Print and shaded views of the part. All mm, measured from the part's lowest x, y and z. Give positions to 0.01 mm unless a question says otherwise; leave off trailing zeros. Write each loop counter-clockwise with the first axis right and the second up, starting at its lowest first coordinate (ties: lowest second). Pieces come first, ordered by that corner, then holes. Notation, with made-up numbers: M 51,-2 L 79,-2 A20 ccw 79,4 Z; hole C 38,18 d1. An arc over 180 degrees is marked long. One line per question, with ' | ' between items. Start each with the question number.
1. Flat gauge pins, fed straight in: pin 1 (2 mm diameter, centred on x = 26.5, y = 117.5, fed in from -Z); pin 2 (6 mm diameter, centred on y = 52, z = 161, fed in from -X); pin 3 (2 mm diameter, centred on y = 272.5, z = 48.5, fed in from -X). Where does each tip first touch, or does it go through?
2. Cut at A-A, the plane x = 10. Write the cut outline in (y, z), then the cut area to 3 significant figures.
3. Wall check: L1, parallel to X at y = 82, z = 153; L2, parallel to Y at x = 90, z = 57.5; L3, parallel to Z at x = 62.5, y = 98. Give the ranges that are in metal, low to high.
4. Pull direction X, two halves, no side cores. Call the marked faces 1, 2 and 3: released by +X, released by -X, zero draft, split by the parting line, or undercut.
5. Cut at D-D, the plane x = 48.5. Write the cut outline in (y, z), then the cut area to 3 significant figures.
6. Cut at B-B, the plane y = 252. Write the cut outline in (x, z).
7. Cut at C-C, the plane y = 144.5. Write the cut outline in (x, z) (1 decimal).
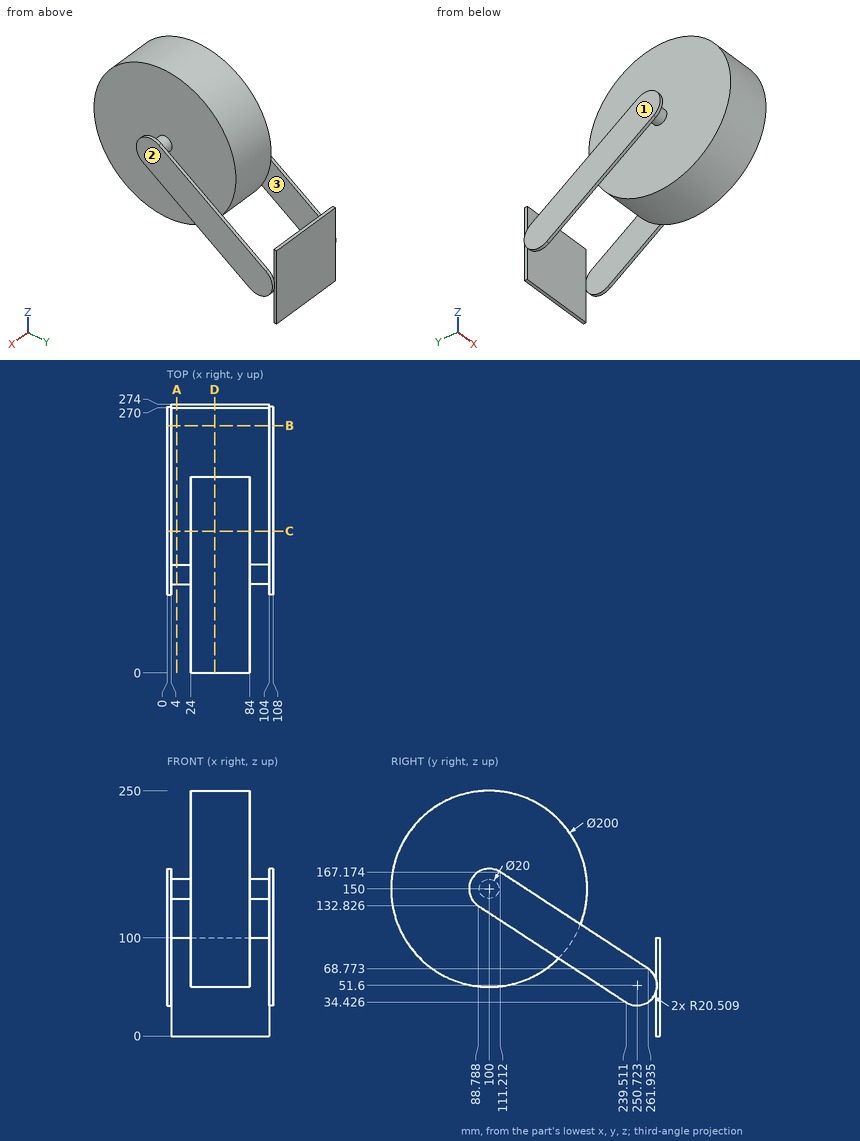
Here are the results:
1) pin 1: z = 51.37 | pin 2: x = 24 | pin 3: x = 4
2) outline: C 100,150 d20; M 270,0 L 274,0 L 274,100 L 270,100 Z | area: 714 mm^2
3) L1: 0 to 4, 24 to 84, 104 to 108 | L2: 270 to 274 | L3: 50.02 to 249.98
4) face 1: released by -X | face 2: released by +X | face 3: undercut
5) outline: C 100,150 d200; M 270,0 L 274,0 L 274,100 L 270,100 Z | area: 31,800 mm^2
6) outline: M 0,31.13 L 4,31.13 L 4,75.26 L 0,75.26 Z; M 104,31.13 L 108,31.13 L 108,75.26 L 104,75.26 Z
7) outline: M 0,96.5 L 4,96.5 L 4,145.4 L 0,145.4 Z; M 24,60.4 L 84,60.4 L 84,239.6 L 24,239.6 Z; M 104,96.5 L 108,96.5 L 108,145.4 L 104,145.4 Z
